Design review of the part built by this model. Coordinates are the model's own, in mm. Give positions to 0.01 mm unless a question says otherwise; leave off trailing zeros. Order: outer loops, then holes, each group sorted by start corner. A loop starts at its lowest first (then second) coordinate and runs counter-clockwise, first axis right, second up. Notation, with made-up numbers: M 76,25.25 L 127,25.25 A15 ccw 127,47.25 Z; hole C 54.5,12.25 d9. An arc over 180 degrees is marked long. Answer as a JSON object with one key per item and string values.
from build123d import *

# Parameters (mm, degrees)
F6_W     = 40
F6_H     = 20
F6_R     = 6
F7_DEPTH = 4
F0_D     = 2
F1_D     = 9
F2_R     = 2
F4_D     = 5.5


with BuildPart() as f7:
    # F6 (on Top) → F7 (new body)
    with BuildSketch(Plane.XY):
        Rectangle(F6_W, F6_H)
        Circle(F6_R, mode=Mode.SUBTRACT)
        Circle(F6_R)
    extrude(amount=F7_DEPTH)

    # F0 (through all)
    with Locations(Plane(origin=(0, 0, 0), x_dir=(1, 0, 0), z_dir=(0, 0, -1))):
        with Locations((0, -6), (-6, 0), (6, 0), (0, 6)):
            Hole(F0_D / 2)

    # F1 (through all)
    with Locations(Plane.XY.offset(4)):
        with Locations((0, 0)):
            Hole(F1_D / 2)

    # F2
    f2_edges = [f7.edges().sort_by_distance(p)[0] for p in [
        (20, 10, 2),
        (20, -10, 2),
        (-20, -10, 2),
        (-20, 10, 2),
    ]]
    fillet(f2_edges, radius=F2_R)

    # F4 (through all)
    with Locations(Plane.XY.offset(4)):
        with Locations((10, 0), (-10, 0)):
            Hole(F4_D / 2)


solid = f7.part
(1) Draft analysis for pull direction X (two halves, no side actions). For faces 1 (the cylindrical face through (0.59, 4.46, 1.97)), 2 (the cylindrical face through (19.4, -9.43, 2.03)), 3 (the cylindrical face through (-19.43, 9.4, 2.03)), state which applies: +X half, -X half, draft (parallel to the pull), parting line (faces both ways), or undercut.
Checked values:
{"face 1": "undercut", "face 2": "+X half", "face 3": "-X half"}
(2) We need section B-B (x = 6). Write out the cut boundary in (y, z), plus the area to 3 significant figures.
Checked values:
{"outline": "M -10,0 L -1,0 L -1,4 L -10,4 Z; M 1,0 L 10,0 L 10,4 L 1,4 Z", "area": "72.0 mm^2"}
(3) To check wall thickness, follow L1, parallel to Y at x = 0, z = 0.8; L2, parallel to Y at x = 6, z = 2.05; L3, parallel to Y at x = 10, z = 1.9. State the ranges of each line that lie inside material, in increasing order. Write a range as from..to.
Checked values:
{"L1": "y = -10..-7, -5..-4.5, 4.5..5, 7..10", "L2": "y = -10..-1, 1..10", "L3": "y = -10..-2.75, 2.75..10"}
(4) We need section C-C (z = 2.3). Write out the cut boundary in (x, y), plus the area to 3 significant figures.
Checked values:
{"outline": "M -20,-8 A2 ccw -18,-10 L 18,-10 A2 ccw 20,-8 L 20,8 A2 ccw 18,10 L -18,10 A2 ccw -20,8 Z; hole C -10,0 d5.5; hole C -6,0 d2; hole C 0,0 d9; hole C 0,-6 d2; hole C 0,6 d2; hole C 6,0 d2; hole C 10,0 d5.5", "area": "673 mm^2"}
(5) We need section A-A (x = 0). Write out the cut boundary in (y, z).
Checked values:
{"outline": "M -10,0 L -7,0 L -7,4 L -10,4 Z; M -5,0 L -4.5,0 L -4.5,4 L -5,4 Z; M 4.5,0 L 5,0 L 5,4 L 4.5,4 Z; M 7,0 L 10,0 L 10,4 L 7,4 Z"}
(6) We need section D-D (y = -6). Write out the cut boundary in (x, z), plus the area to 3 significant figures.
Checked values:
{"outline": "M -20,0 L -1,0 L -1,4 L -20,4 Z; M 1,0 L 20,0 L 20,4 L 1,4 Z", "area": "152 mm^2"}
